Verification items for the finished model (mm, model axes). A direction names the side the tool comes from. Round coordinates to 2 decimals unless told otherwise and drop trailing zeros. Loops run counter-clockwise (first coordinate to the right, second up) from the corner with the lowest first, then second, coordinate; pieces in that order, holes last. Notation, with made-up numbers: (54.5, -17) -> (70.5, -17) arc R14 cw to (70.5, -3) -> close; hole circle Ø11 at (47.25, -10). An arc over 180 degrees is marked (long way). Write item = value, one per line.
```python
from build123d import *

# Parameters (mm, degrees)
SKETCH_W            = 20
SKETCH_H            = 25
PAD_DEPTH           = 6
SKETCH001_R         = 1.7
POCKET_DEPTH        = 10
SKETCH002_W         = 2
SKETCH002_H         = 4
POCKET001_DEPTH     = 25
LINEARPATTERN_COUNT = 8
LINEARPATTERN_PITCH = 3
SKETCH003_R         = 3
POCKET002_DEPTH     = 4.5


with BuildPart() as part:
    # Sketch → Pad (new body)
    with BuildSketch(Plane.XZ):
        Rectangle(SKETCH_W, SKETCH_H)
    extrude(amount=PAD_DEPTH)

    # Sketch001 (on Face6 of Pad) → Pocket (cut)
    with BuildSketch(Plane.XZ.offset(6)):
        with Locations((0, 2.5)):
            Circle(SKETCH001_R)
    extrude(amount=-POCKET_DEPTH, mode=Mode.SUBTRACT)

    # Sketch002 (on Face2 of Pocket) → Pocket001 (cut)
    with BuildSketch(Plane(origin=(-10, 0, 0), x_dir=(0, 0, -1), z_dir=(-1, 0, 0))):
        with Locations((-10.5, 4)):
            Rectangle(SKETCH002_W, SKETCH002_H)
    pocket001 = extrude(amount=-POCKET001_DEPTH, mode=Mode.SUBTRACT)

    # LinearPattern: Pocket001 ×8
    with Locations(*[(0, 0, -i * LINEARPATTERN_PITCH) for i in range(1, LINEARPATTERN_COUNT)]):
        add(pocket001, mode=Mode.SUBTRACT)

    # Sketch003 (on Face40 of LinearPattern) → Pocket002 (cut)
    with BuildSketch(Plane.XZ.offset(6)):
        with Locations((0, 2.5)):
            Circle(SKETCH003_R)
    extrude(amount=-POCKET002_DEPTH, mode=Mode.SUBTRACT)


with BuildPart() as part_1:
    # Body002 placement: moved
    add(part.part.moved(Location((0, 100, 0))))


solid = part_1.part
```
(1) Sectioned sample at A-A, the plane y = 98.85. Record the cut outline in (x, z), and give its area (3 significant figures).
Filled sheet:
outline = (-10, -12.5) -> (10, -12.5) -> (10, 12.5) -> (-10, 12.5) -> close; hole circle Ø3.4 at (0, 2.5)
area = 491 mm2
(2) Draft check along Z on faces 4 (the face through (0, 97, -12.5)), 5 (the face through (-6, 96, 3.5)), 6 (the face through (0, 94, -3)). Enter one of: released by +Z, released by -Z, zero draft, split by the parting line, or undercut.
Filled sheet:
face_4 = released by -Z
face_5 = undercut
face_6 = zero draft
(3) Set-up check for faces 1 (the face through (1.384, 96.218, -0.162)), 2 (the face through (-0.221, 99.239, 4.186)), 3 (the face through (0, 96, -6.5)): record each of +Z, -Z, +X, -X, +Y, -Y from which the full face is reachable in a straight line by a thin tool's end or side.
Filled sheet:
face_1 = -Y
face_2 = +Y, -Y
face_3 = +X, -X, -Y
(4) Material ranges on probe 1 along Z at (x, y) = (0, 99.4); probe 2 along Y at (x, z) = (8.75, -10), recorded low to high. Write a range as from..to.
Filled sheet:
probe_1 = -12.5..0.8, 4.2..12.5
probe_2 = 98..100
(5) Go/stop test with a flat-tipped pin: pin 1 Ø3 at (x, z) = (-1.5, 2) entering from -Y. Record where the tip stops, or that it passes through.
Filled sheet:
pin_1 = 98
